The model under review builds one solid part; all positions refer to its coordinate system, in mm. A direction names the side the tool comes from. Coordinates: 2 decimals unless noted, no trailing zeros. Write each loop counter-clockwise with the first axis right and the second up, starting at its lowest first coordinate (ties: lowest second). Pieces come first, ordered by that corner, then holes. Notation, with made-up numbers: M -23,4.25 L -4,4.25 A10 cw -4,14.25 Z; hole C 74.5,-6.5 d5. An arc over 180 degrees is marked long. Answer as a JSON object with one key per item and string values.
```python
from build123d import *

# Parameters (mm, degrees)
SKETCH1_W           = 29.464
SKETCH1_H           = 19.05
BOSS_EXTRUDE1_DEPTH = 355.6
SKETCH2_W           = 29.464
SKETCH2_H           = 25.4
BOSS_EXTRUDE2_DEPTH = 50.8


with BuildPart() as part:
    # Sketch1 → Boss-Extrude1 (new, symmetric)
    with BuildSketch(Plane.XY):
        with Locations((0, -9.525)):
            Rectangle(SKETCH1_W, SKETCH1_H)
    extrude(amount=BOSS_EXTRUDE1_DEPTH, both=True)

    # Sketch2 → Boss-Extrude2 (add)
    with BuildSketch(Plane(origin=(0, 0, 0), x_dir=(1, 0, 0), z_dir=(0, 1, 0))):
        with Locations((0, 63.5)):
            Rectangle(SKETCH2_W, SKETCH2_H)
        with Locations((0, -63.5)):
            Rectangle(SKETCH2_W, SKETCH2_H)
    extrude(amount=BOSS_EXTRUDE2_DEPTH)


solid = part.part
```
(1) For pin 1 Ø12 at (x, y) = (6, 30) entering from -Z; pin 2 Ø1.5 at (x, y) = (4.5, 17) entering from +Z; pin 3 Ø9 at (x, z) = (2, -224) entering from +Y, all flat-tipped, find the tip position at first contact; note any pin that passes through.
Results list:
{"pin 1": "z = -76.2", "pin 2": "z = 76.2", "pin 3": "y = 0"}
(2) For faces 5 (the face through (0, 0, 218)), 6 (the face through (0, 25, -76.2)), 7 (the face through (0, 0, 1)), list the 3-axis set-ups (+Z, -Z, +X, -X, +Y, -Y) from which the entire face can be reached by the end or side of a thin tool; tool diameter is ignored.
Results list:
{"face 5": "+Z, +X, -X, +Y", "face 6": "-Z, +X, -X, +Y", "face 7": "+X, -X, +Y"}
(3) Wall thickness on line 1 along Z through (x, y) = (0.25, 9.5); line 2 along Y through (x, z) = (-2.5, -132): over which ranges is each line inside the solid? List them lowest first. Write a range as from..to.
Results list:
{"line 1": "-76.2..-50.8, 50.8..76.2", "line 2": "-19.05..0"}
(4) Add section C-C on z = -208. Give the boundary of the cut face in (x, y), and give its area (3 significant figures).
Results list:
{"outline": "M -14.73,-19.05 L 14.73,-19.05 L 14.73,0 L -14.73,0 Z", "area": "561 mm²"}
(5) Add section B-B on x = -9.5. Give the boundary of the cut face in (y, z).
Results list:
{"outline": "M -19.05,-355.6 L 0,-355.6 L 0,-76.2 L 50.8,-76.2 L 50.8,-50.8 L 0,-50.8 L 0,50.8 L 50.8,50.8 L 50.8,76.2 L 0,76.2 L 0,355.6 L -19.05,355.6 Z"}
(6) Add section A-A on y = 31. Give the boundary of the cut face in (x, z), and give its area (3 significant figures).
Results list:
{"outline": "M -14.73,-76.2 L 14.73,-76.2 L 14.73,-50.8 L -14.73,-50.8 Z; M -14.73,50.8 L 14.73,50.8 L 14.73,76.2 L -14.73,76.2 Z", "area": "1,500 mm²"}
(7) Draft analysis for pull direction Z (two halves, no side actions). For faces 1 (the face through (0, 25, 76.2)), 2 (the face through (0, 50.8, 63)), 3 (the face through (0, 25, -50.8)), 4 (the face through (0, 25, 50.8)), state which applies: released by +Z, released by -Z, zero draft, split by the parting line, or undercut.
Results list:
{"face 1": "released by +Z", "face 2": "zero draft", "face 3": "undercut", "face 4": "undercut"}
